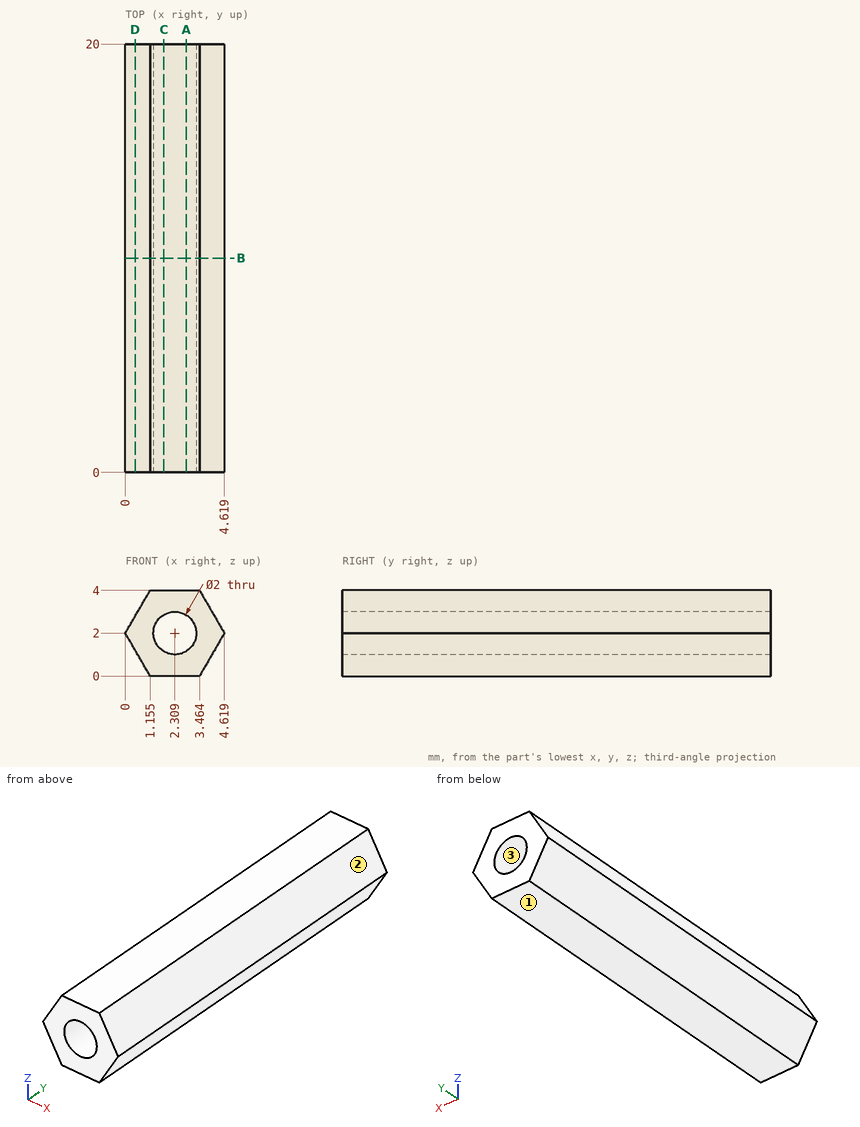
For this review, use the dimensioned drawing (mm, ordinates from the lowest corner) and the shaded views. Coordinates: 2 decimals unless noted, no trailing zeros. Write each loop counter-clockwise with the first axis right and the second up, starting at its lowest first coordinate (ties: lowest second). Pieces come first, ordered by that corner, then holes. Notation, with made-up numbers: (-29, 73.5) - (23, 73.5) arc R12 cw to (23, 93.5) - close; hole circle Ø2 at (-4, 82). An arc over 180 degrees is marked (long way). Answer as a JSON object with one key per item and string values. Group by question number.
1. Add section B-B (y = 10). Give the boundary of the cut face in (x, z) (1 decimal), plus the area to 3 significant figures.
2. To check wall thickness, follow probe 1 along Z at (x, y) = (1.6, 8.5) (1 decimal); probe 2 along Z at (x, y) = (3.1, 8.75) (1 decimal); probe 3 along X at (y, z) = (17.5, 2.8) (1 decimal). State the ranges of each line that lie inside material, in increasing order.
3. Add section A-A (x = 2.85). Give the boundary of the cut face in (y, z).
4. Mouldability with a two-part tool opening along X and no side actions: class the marked faces 1, 2 and 3 as pulls with the +X half, pulls with the -X half, needs draft (parallel to the pull), parting line crosses it, or undercut.
5. Add section C-C (x = 1.8). Give the boundary of the cut face in (y, z).
6. Add section D-D (x = 0.45). Give the boundary of the cut face in (y, z).
Findings:
{
 "1": {"outline": "(0, 2) - (1.2, 0) - (3.5, 0) - (4.6, 2) - (3.5, 4) - (1.2, 4) - close; hole circle Ø2 at (2.3, 2)", "area": "10.7 mm²"},
 "2": {"probe 1": "0 to 1.3, 2.7 to 4", "probe 2": "0 to 1.4, 2.6 to 4", "probe 3": "0.5 to 1.7, 2.9 to 4.2"},
 "3": {"outline": "(0, 0) - (20, 0) - (20, 1.16) - (0, 1.16) - close; (0, 2.84) - (20, 2.84) - (20, 4) - (0, 4) - close"},
 "4": {"face 1": "needs draft", "face 2": "pulls with the +X half", "face 3": "undercut"},
 "5": {"outline": "(0, 0) - (20, 0) - (20, 1.14) - (0, 1.14) - close; (0, 2.86) - (20, 2.86) - (20, 4) - (0, 4) - close"},
 "6": {"outline": "(0, 1.22) - (20, 1.22) - (20, 2.78) - (0, 2.78) - close"}
}
